Verification items for the finished model (mm, model axes). A direction names the side the tool comes from. Give positions to 0.01 mm unless a question says otherwise; leave off trailing zeros. Order: outer loops, then holes, each group sorted by start corner. A loop starts at its lowest first (then second) coordinate and runs counter-clockwise, first axis right, second up. Notation, with made-up numbers: (-12.5, 85.25) -> (27.5, 85.25) arc R33 cw to (27.5, 113.25) -> close; hole circle Ø8 at (-2, -30.75). An arc over 180 degrees is marked (long way). One line per question, with ' | ' between items. Start each with the question number.
Q1. Mould release check, pull along X, two halves, no side actions. Record for faces 1 (the flat face through (-2, 914.4, 18)), 2 (the flat face through (-19.05, 451, 0)), 3 (the flat face through (19.05, 451, 0)), 4 (the flat face through (-17.462, 451, 0)): released by +X, released by -X, zero draft, split by the parting line, or undercut.
Q2. Access from +Z, -Z, +X, -X, +Y, -Y to the whole of each face (thin tool, end or side, straight path). Record for faces 5 (the flat face through (0, 451, -17.462)), 6 (the flat face through (0, 451, 19.05)).
Q3. Section check B-B on y = 31.75. Record the cut outline in (x, z), plus the area to 3 significant figures.
Q4. Material ranges on probe 1 along Y at (x, z) = (0, -17.85); probe 2 along X at (y, z) = (152, 1), recorded low to high. Write a range as [from, to].
Q5. Section check A-A on y = 167. Record the cut outline in (x, z).
Q6. Go/stop test with flat-tipped pins: pin 1 (6 mm diameter, centred on y = 114.3, z = 0, fed in from -X); pin 2 (4 mm diameter, centred on x = 0, y = 114.3, fed in from +Z). Record where each tip stops, or that it passes through.
from build123d import *

# Parameters (mm, degrees)
SKETCH1_W           = 38.1
SKETCH1_H           = 38.1
SKETCH1_W_2         = 34.925
SKETCH1_H_2         = 34.925
BOSS_EXTRUDE1_DEPTH = 914.4
SKETCH2_R           = 2.5527
CUT_EXTRUDE1_DEPTH  = 916.391649787
SKETCH3_R           = 2.5527
CUT_EXTRUDE2_DEPTH  = 916.391649787
SKETCH4_R           = 14.2875
SKETCH4_R_2         = 2.5527
CUT_EXTRUDE3_DEPTH  = 916.391649787


with BuildPart() as part:
    # Sketch1 → Boss-Extrude1 (new body)
    with BuildSketch(Plane(origin=(0, 0, 0), x_dir=(1, 0, 0), z_dir=(0, 1, 0))):
        Rectangle(SKETCH1_W, SKETCH1_H)
        Rectangle(SKETCH1_W_2, SKETCH1_H_2, mode=Mode.SUBTRACT)
    extrude(amount=BOSS_EXTRUDE1_DEPTH)

    # Sketch2 → Cut-Extrude1 (cut, through all)
    with BuildSketch(Plane.XY.offset(19.05)):
        with Locations((0, 76.2)):
            Circle(SKETCH2_R)
        with Locations((0, 95.25)):
            Circle(SKETCH2_R)
        with Locations((0, 114.3)):
            Circle(SKETCH2_R)
        with Locations((0, 133.35)):
            Circle(SKETCH2_R)
        with Locations((9.525, 104.775)):
            Circle(SKETCH2_R)
    extrude(amount=-CUT_EXTRUDE1_DEPTH, mode=Mode.SUBTRACT)

    # Sketch3 → Cut-Extrude2 (cut, through all)
    with BuildSketch(Plane(origin=(19.05, 0, 0), x_dir=(0, 0, -1), z_dir=(1, 0, 0))):
        with Locations((0, 76.2)):
            Circle(SKETCH3_R)
        with Locations((0, 95.25)):
            Circle(SKETCH3_R)
        with Locations((0, 114.3)):
            Circle(SKETCH3_R)
        with Locations((-9.525, 225.425)):
            Circle(SKETCH3_R)
        with Locations((-9.525, 206.375)):
            Circle(SKETCH3_R)
        with Locations((-9.525, 187.325)):
            Circle(SKETCH3_R)
        with Locations((9.525, 187.325)):
            Circle(SKETCH3_R)
        with Locations((9.525, 206.375)):
            Circle(SKETCH3_R)
        with Locations((9.525, 225.425)):
            Circle(SKETCH3_R)
        with Locations((0, 904.875)):
            Circle(SKETCH3_R)
        with Locations((0, 885.825)):
            Circle(SKETCH3_R)
    extrude(amount=-CUT_EXTRUDE2_DEPTH, mode=Mode.SUBTRACT)

    # Sketch4 → Cut-Extrude3 (cut, through all)
    with BuildSketch(Plane(origin=(19.05, 0, 0), x_dir=(0, 0, -1), z_dir=(1, 0, 0))):
        with Locations((0, 31.75)):
            Circle(SKETCH4_R)
        with Locations((-11.90625, 52.372229928)):
            Circle(SKETCH4_R_2)
        with Locations((11.90625, 52.372229928)):
            Circle(SKETCH4_R_2)
        with Locations((11.90625, 11.127770072)):
            Circle(SKETCH4_R_2)
        with Locations((-11.90625, 11.127770072)):
            Circle(SKETCH4_R_2)
    extrude(amount=-CUT_EXTRUDE3_DEPTH, mode=Mode.SUBTRACT)


solid = part.part
Filled in:
1) face 1: zero draft | face 2: released by -X | face 3: released by +X | face 4: undercut
2) face 5: +Y, -Y | face 6: +Z, +X, -X, +Y, -Y
3) outline: (-19.05, -19.05) -> (19.05, -19.05) -> (19.05, -14.29) -> (17.46, -14.29) -> (17.46, -17.46) -> (-17.46, -17.46) -> (-17.46, -14.29) -> (-19.05, -14.29) -> close; (-19.05, 14.29) -> (-17.46, 14.29) -> (-17.46, 17.46) -> (17.46, 17.46) -> (17.46, 14.29) -> (19.05, 14.29) -> (19.05, 19.05) -> (-19.05, 19.05) -> close | area: 141 mm²
4) probe 1: [0, 73.65], [78.75, 92.7], [97.8, 111.75], [116.85, 130.8], [135.9, 914.4] | probe 2: [-19.05, -17.46], [17.46, 19.05]
5) outline: (-19.05, -19.05) -> (19.05, -19.05) -> (19.05, 19.05) -> (-19.05, 19.05) -> close; hole (-17.46, -17.46) -> (17.46, -17.46) -> (17.46, 17.46) -> (-17.46, 17.46) -> close
6) pin 1: x = -19.05 | pin 2: through
